Work out the finished part from the listing and answer in its coordinate system (mm). Face numbers are marked on the shaded views. Round coordinates to 2 decimals unless told otherwise and drop trailing zeros. Loops run counter-clockwise (first coordinate to the right, second up) from the corner with the lowest first, then second, coordinate; pieces in that order, holes last. Notation, with made-up numbers: M -26,-15 L -3,-15 A10 ccw -3,4 Z; hole C -6.5,-20.5 d8. An arc over 180 degrees is marked long. One line per item, written item: value.
```python
from build123d import *

# Parameters (mm, degrees)
F0_W     = 10
F0_H     = 170
F1_DEPTH = 37.5
F2_W     = 65
F2_H     = 4.9
F3_DEPTH = 10
F4_W     = 75
F4_H     = 170
F4_W_2   = 65
F4_H_2   = 154.9
F5_DEPTH = 50
F6_W     = 75
F6_H     = 170
F7_DEPTH = 5
F8_W     = 25
F8_H     = 50
F9_DEPTH = 5


with BuildPart() as f1:
    # F0 (on Right) → F1 (new body, symmetric)
    with BuildSketch(Plane.YZ):
        with Locations((-36.757313, -17.352806)):
            Rectangle(F0_W, F0_H)
    extrude(amount=F1_DEPTH, both=True)

    # F2 (on face) → F3 (cut, through all)
    with BuildSketch(Plane.XZ.offset(41.757313)):
        with Locations((0, 60.197194)):
            Rectangle(F2_W, F2_H)
        with Locations((0, 50.197194)):
            Rectangle(F2_W, F2_H)
        with Locations((0, 40.197194)):
            Rectangle(F2_W, F2_H)
        with Locations((0, 30.197194)):
            Rectangle(F2_W, F2_H)
        with Locations((0, 20.197194)):
            Rectangle(F2_W, F2_H)
        with Locations((0, 10.197194)):
            Rectangle(F2_W, F2_H)
        with Locations((0, 0.197194)):
            Rectangle(F2_W, F2_H)
        with Locations((0, -9.802806)):
            Rectangle(F2_W, F2_H)
        with Locations((0, -19.802806)):
            Rectangle(F2_W, F2_H)
        with Locations((0, -29.802806)):
            Rectangle(F2_W, F2_H)
        with Locations((0, -39.802806)):
            Rectangle(F2_W, F2_H)
        with Locations((0, -49.802806)):
            Rectangle(F2_W, F2_H)
        with Locations((0, -59.802806)):
            Rectangle(F2_W, F2_H)
        with Locations((0, -69.802806)):
            Rectangle(F2_W, F2_H)
        with Locations((0, -79.802806)):
            Rectangle(F2_W, F2_H)
        with Locations((0, -89.802806)):
            Rectangle(F2_W, F2_H)
    extrude(amount=-F3_DEPTH, mode=Mode.SUBTRACT)

    # F4 (on face) → F5 (join)
    with BuildSketch(Plane(origin=(0, -31.757313, 0), x_dir=(-1, 0, 0), z_dir=(0, 1, 0))):
        with Locations((0, -17.352806)):
            Rectangle(F4_W, F4_H)
        with Locations((0, -14.802806)):
            Rectangle(F4_W_2, F4_H_2, mode=Mode.SUBTRACT)
    extrude(amount=F5_DEPTH)

    # F6 (on face) → F7 (join)
    with BuildSketch(Plane(origin=(0, 18.242687, 0), x_dir=(-1, 0, 0), z_dir=(0, 1, 0))):
        with Locations((0, -17.352806)):
            Rectangle(F6_W, F6_H)
    extrude(amount=F7_DEPTH)

    # F8 (on face) → F9 (cut, through all)
    with BuildSketch(Plane(origin=(0, 23.242687, 0), x_dir=(-1, 0, 0), z_dir=(0, 1, 0))):
        with Locations((0, -17.352806)):
            Rectangle(F8_W, F8_H)
    extrude(amount=-F9_DEPTH, mode=Mode.SUBTRACT)


solid = f1.part
```
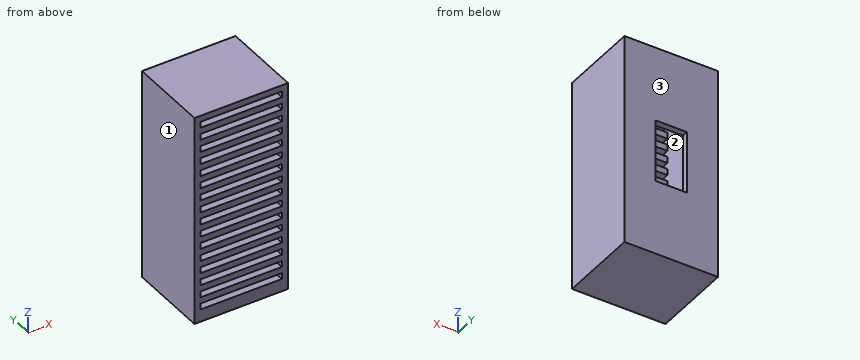
1) The mould has two halves that part along Y. Classify the marked faces 1, 2 and 3: +Y half, -Y half, draft (parallel to the pull), parting line (faces both ways), or undercut.
Check values:
face 1: draft
face 2: undercut
face 3: +Y half
2) Find section B-B (z = -80). Give the vertices of the cut face in (x, y).
Check values:
outline: M -37.5,-41.76 L -32.5,-41.76 L -32.5,18.24 L 32.5,18.24 L 32.5,-41.76 L 37.5,-41.76 L 37.5,23.24 L -37.5,23.24 Z
3) Find section A-A (y = 3.5). Give the vertices of the cut face in (x, z).
Check values:
outline: M -37.5,-102.35 L 37.5,-102.35 L 37.5,67.65 L -37.5,67.65 Z; hole M -32.5,-92.25 L 32.5,-92.25 L 32.5,62.65 L -32.5,62.65 Z
4) Find the intervals of material crossed by probe 1 along X at (y, z) = (16.5, 25); probe 2 along Z at (x, y) = (24, -9); probe 3 along Y at (x, z) = (29, 57), in increasing order. Write a range as from..to.
Check values:
probe 1: -37.5..-32.5, 32.5..37.5
probe 2: -102.35..-92.25, 62.65..67.65
probe 3: -41.76..-31.76, 18.24..23.24
5) This flat-tipped pin is pushed along its axis until it touches: pin 1 (19.5 mm diameter, centred on x = -13.5, z = -30.5, fed in from -Y). Where does it stop, or does it pass through?
Check values:
pin 1: y = -41.76
6) Find section C-C (x = 16.5). Give the number of separate pieces and of enclosed holes in the cut face, then the cut area to 3 significant figures.
Check values:
separate pieces: 16
enclosed holes: 0
area: 2,520 mm2
